The listing builds one solid part. Answer for the finished solid, in the listing's coordinates (mm). A direction names the side the tool comes from. Give positions to 0.01 mm unless a question says otherwise; leave off trailing zeros. Write each loop counter-clockwise with the first axis right and the second up, starting at its lowest first coordinate (ties: lowest second). Pieces come first, ordered by that corner, then holes.
Autodesk Inventor part; units mm, degrees
ref_plane "YZ Plane" through (0, 0, 0) normal (1, 0, 0) x (0, 1, 0)
ref_plane "XZ Plane" through (0, 0, 0) normal (0, 1, 0) x (-1, 0, 0)
ref_plane "XY Plane" through (0, 0, 0) normal (0, 0, 1) x (1, 0, 0)
sketch "Sketch1" plane through (0, 0, 0) normal (0, 0, 1) x (1, 0, 0)
  line L0 (2.3725, 4.0488) -> (4.6926, -0.0303)
  line L1 (4.6926, -0.0303) -> (2.3201, -4.0791)
  line L2 (2.3201, -4.0791) -> (-2.3725, -4.0488)
  line L3 (-2.3725, -4.0488) -> (-4.6926, 0.0303)
  line L4 (-4.6926, 0.0303) -> (-2.3201, 4.0791)
  line L5 (-2.3201, 4.0791) -> (2.3725, 4.0488)
  point P0 (0, 0)
  point P1 (0, 0)
  dimension "d0" = 8.128
extrude "Extrusion1" add sketch "Sketch1" along normal blind 1.27
sketch "Sketch2" plane through (0, 0, 1.27) normal (0, 0, 1) x (1, 0, 0)
  circle A0 centre (0, 0) radius 3.175
  dimension "d3" = 6.35
extrude "Extrusion2" add sketch "Sketch2" along normal blind 11.43
thread "Thread1"
sketch "Sketch3" plane through (0, 0, 12.7) normal (0, 0, 1) x (1, 0, 0)
  circle A0 centre (0, 0) radius 3.175
  circle A1 centre (0, 0) radius 2.667
  dimension "d9" = 0.508
extrude "Extrusion3" cut sketch "Sketch3" against normal blind 2.54 contours A1
sketch "Sketch4" plane through (0, 0, 10.16) normal (0, 0, 1) x (1, 0, 0)
  circle A0 centre (0, 0) radius 2.667
  circle A1 centre (0, 0) radius 0.4071
extrude "Extrusion4" cut sketch "Sketch4" against normal blind 2.54 contours A1
sketch "Sketch5" plane through (0, 0, 0) normal (0, 0, -1) x (-1, 0, 0)
  circle A0 centre (0, 0) radius 1.905
  dimension "d14" = 3.81
extrude "Extrusion5" add sketch "Sketch5" along normal blind 12.7
properties part number "sma_female_bulkhead" material "Gold"
Item 1: Determine the mould class of faces 1 (the face through (-3.52, 2.03, 0.63)), 2 (the face through (3.52, -2.03, 0.63)), 3 (the face through (-0.088, -0.397, 8.908)), 4 (the face through (0, 0, 7.62)) for opening direction X: pulls with the +X half, pulls with the -X half, needs draft (parallel to the pull), parting line crosses it, or undercut.
Conclusion:
face 1: pulls with the -X half
face 2: pulls with the +X half
face 3: undercut
face 4: undercut
Item 2: A cutting plane is placed at D-D, the plane z = -10.5. Give the vertices of the cut face in (x, y) (3 decimals).
Conclusion:
outline: circle Ø3.81 at (0, 0)
Item 3: Each of these flat-tipped pins is pushed along its axis until it touches: P1, Ø2, axis at y = 1, z = 8, coming from the -X side (3 decimals); P2, Ø3, axis at x = 0, y = 0, coming from the +Z side; P3, Ø1.5, axis at y = -0.5, z = -6, coming from the -X side (3 decimals); P4, Ø1.5, axis at x = 2.5, y = 0, coming from the -Z side. Where does it stop, or does it pass through?
Conclusion:
P1: stops at x = -3.175
P2: stops at z = 10.16
P3: stops at x = -1.905
P4: stops at z = -12.7
Item 4: A cutting plane is placed at C-C, the plane y = -1.25. Give the vertices of the cut face in (x, z).
Conclusion:
outline: (-3.96, 0) - (-1.44, 0) - (-1.44, -12.7) - (1.44, -12.7) - (1.44, 0) - (3.98, 0) - (3.98, 1.27) - (2.92, 1.27) - (2.92, 12.7) - (2.36, 12.7) - (2.36, 10.16) - (-2.36, 10.16) - (-2.36, 12.7) - (-2.92, 12.7) - (-2.92, 1.27) - (-3.96, 1.27) - close
Item 5: Which of the six approach directions +Z, -Z, +X, -X, +Y, -Y give full straight-line access (tool end or side, diameter ignored) to faces 5 (the face through (3.516, 2.038, 0.626)), 6 (the face through (1.231, -2.366, 11.448)), 7 (the face through (1, 2, 0))?
Conclusion:
face 5: +Z, -Z, +X, +Y
face 6: +Z
face 7: -Z
Item 6: Consider probe 1 along Y at (x, z) = (0, 8.7) (3 decimals); probe 2 along Y at (x, z) = (0, 10.25) (3 decimals); probe 3 along Z at (x, y) = (3, 1.25). Determine where each line is inside the solid, lowest interval first.
Conclusion:
probe 1: y = -3.175 to -0.407, 0.407 to 3.175
probe 2: y = -3.175 to -2.667, 2.667 to 3.175
probe 3: z = 0 to 1.27
Item 7: A cutting plane is placed at B-B, the plane z = 10.5. Give the vertices of the cut face in (x, y) (3 decimals), plus the area to 3 significant figures.
Conclusion:
outline: circle Ø6.35 at (0, 0); hole circle Ø5.334 at (0, 0)
area: 9.32 mm2
Item 8: A cutting plane is placed at A-A, the plane x = -1. Give the vertices of the cut face in (y, z), plus the area to 3 significant figures.
Conclusion:
outline: (-4.06, 0) - (-1.62, 0) - (-1.62, -12.7) - (1.62, -12.7) - (1.62, 0) - (4.07, 0) - (4.07, 1.27) - (3.01, 1.27) - (3.01, 12.7) - (2.47, 12.7) - (2.47, 10.16) - (-2.47, 10.16) - (-2.47, 12.7) - (-3.01, 12.7) - (-3.01, 1.27) - (-4.06, 1.27) - close
area: 108 mm2
